from build123d import *

# Parameters (mm, degrees)
F0_W     = 400
F0_H     = 25
F2_R     = 20
F3_DEPTH = 30
F4_DEPTH = 30


with BuildPart() as f1:
    # F0 (on Front) → F1 (revolve)
    with BuildSketch(Plane.XZ):
        with Locations((200, 12.5)):
            Rectangle(F0_W, F0_H)
    revolve(axis=Axis((200, 0, 0), (-1, 0, 0)))

    # F2 (on Front) → F3 (join, symmetric)
    with BuildSketch(Plane.XZ):
        with BuildLine():
            Line((26.457513, 30), (-26.457513, 30))
            ThreePointArc((-26.457513, 30), (-40, 0), (-26.457513, -30))
            Line((-26.457513, -30), (26.457513, -30))
            ThreePointArc((26.457513, -30), (40, 0), (26.457513, 30))
        make_face()
        Circle(F2_R, mode=Mode.SUBTRACT)
        Circle(F2_R)
    extrude(amount=F3_DEPTH, both=True)

    # F2 (on Front) → F4 (cut, symmetric)
    with BuildSketch(Plane.XZ):
        Circle(F2_R)
    extrude(amount=F4_DEPTH, both=True, mode=Mode.SUBTRACT)


solid = f1.part
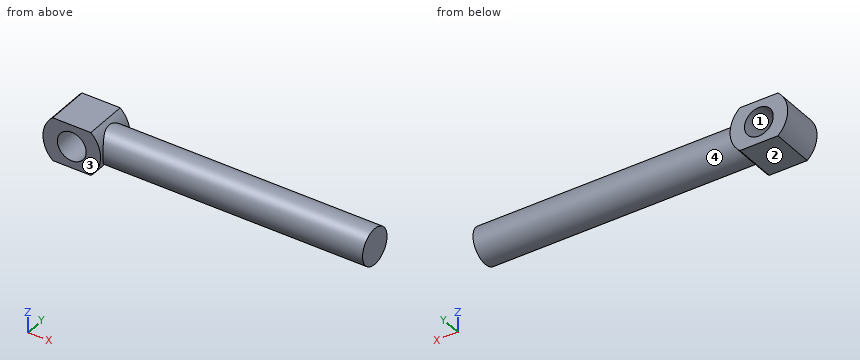
Model file for the job. Use its own axes, mm. Face numbers are marked on the shaded views. Round coordinates to 2 decimals unless told otherwise and drop trailing zeros. Order: outer loops, then holes, each group sorted by start corner. A loop starts at its lowest first (then second) coordinate and runs counter-clockwise, first axis right, second up. Notation, with made-up numbers: M 10,-24 L 20,-24 A16 cw 20,-7 Z; hole C 64.25,3.25 d8. An arc over 180 degrees is marked long. Write each question's results on one line, items separated by ' | '. Start each with the question number.
(1) Probe probe 1 along X at (y, z) = (-27.5, 1.5); probe 2 along Z at (x, y) = (0, -11); probe 3 along Y at (x, z) = (357, -15). List the from-to ranges inside material, lowest first. Write a range as from..to.
(2) Saw through at C-C, the plane x = -12. Give the cut face in (y, z), then the cut area to 3 significant figures.
(3) Saw through at D-D, the plane x = 156.5. Give the cut face in (y, z).
(4) Saw through at A-A, the plane z = 0. Give the cut face in (x, y).
(5) Drop flat-ended pins along their axis: pin 1 (3 mm diameter, centred on x = 164, z = -22, fed in from +Y); pin 2 (2 mm diameter, centred on y = 5, z = 19, fed in from -X); pin 3 (4 mm diameter, centred on x = 220.5, y = 15, fed in from -Z). Give the stop position or say it passes through.
(6) Saw through at B-B, the plane y = 0. Give the cut face in (x, z), then the cut area to 3 significant figures.
(7) Two-plate mould, pull along Z, no slides. Class the marked faces 1, 2, 3 and 4: pulls with the +Z half, pulls with the -Z half, needs draft (parallel to the pull), parting line crosses it, or undercut.
Established:
1) probe 1: x = -39.97..-19.94, 19.94..39.97 | probe 2: z = -30..-20, 20..30 | probe 3: y = -20..20
2) outline: M -30,-30 L 30,-30 L 30,-16 L -30,-16 Z; M -30,16 L 30,16 L 30,30 L -30,30 Z | area: 1,680 mm^2
3) outline: C 0,0 d50
4) outline: M -40,-30 L -20,-30 L -20,30 L -40,30 Z; M 20,-30 L 40,-30 L 40,-25 L 400,-25 L 400,25 L 40,25 L 40,30 L 20,30 Z
5) pin 1: stops at y = 14.31 | pin 2: stops at x = -35.72 | pin 3: stops at z = -21.35
6) outline: M -26.46,-30 L 26.46,-30 A40 ccw 31.22,-25 L 400,-25 L 400,25 L 31.22,25 A40 ccw 26.46,30 L -26.46,30 A40 ccw Z; hole C 0,0 d40 | area: 21,200 mm^2
7) face 1: undercut | face 2: pulls with the -Z half | face 3: needs draft | face 4: parting line crosses it
